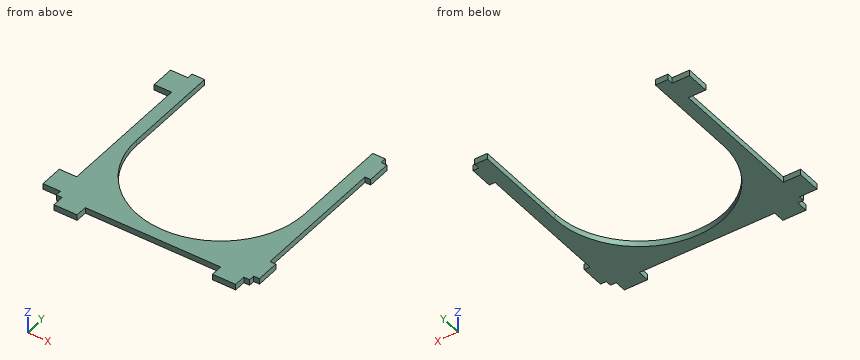
```python
from build123d import *

# Parameters (mm, degrees)
CROQUIS1_W              = 100
CROQUIS1_H              = 100
CROQUIS1_R              = 43.5
SALIENTE_EXTRUIR1_DEPTH = 3
CROQUIS2_W              = 12
CROQUIS2_H              = 6
CROQUIS2_W_2            = 9
CROQUIS2_H_2            = 12
CROQUIS2_W_3            = 3
SALIENTE_EXTRUIR2_DEPTH = 3
CROQUIS3_W              = 87
CROQUIS3_H              = 50
CORTAR_EXTRUIR1_DEPTH   = 10


with BuildPart() as part:
    # Croquis1 → Saliente-Extruir1 (new body)
    with BuildSketch(Plane.XY):
        Rectangle(CROQUIS1_W, CROQUIS1_H)
        Circle(CROQUIS1_R, mode=Mode.SUBTRACT)
    extrude(amount=SALIENTE_EXTRUIR1_DEPTH)

    # Croquis2 → Saliente-Extruir2 (add)
    with BuildSketch(Plane.XY.offset(3)):
        with Locations((-41, -53)):
            Rectangle(CROQUIS2_W, CROQUIS2_H)
        with Locations((41, -53)):
            Rectangle(CROQUIS2_W, CROQUIS2_H)
        with Locations((-54.5, -41)):
            Rectangle(CROQUIS2_W_2, CROQUIS2_H_2)
        with Locations((51.5, -41)):
            Rectangle(CROQUIS2_W_3, CROQUIS2_H_2)
        with Locations((51.5, 41)):
            Rectangle(CROQUIS2_W_3, CROQUIS2_H_2)
        with Locations((-54.5, 41)):
            Rectangle(CROQUIS2_W_2, CROQUIS2_H_2)
    extrude(amount=-SALIENTE_EXTRUIR2_DEPTH)

    # Croquis3 → Cortar-Extruir1 (cut)
    with BuildSketch(Plane.XY.offset(3)):
        with Locations((0, 25)):
            Rectangle(CROQUIS3_W, CROQUIS3_H)
    extrude(amount=-CORTAR_EXTRUIR1_DEPTH, mode=Mode.SUBTRACT)


solid = part.part
```
Geometry: final body of the model. Coordinates: model frame, mm. Round coordinates to 2 decimals unless told otherwise and drop trailing zeros. Order: outer loops, then holes, each group sorted by start corner. A loop starts at its lowest first (then second) coordinate and runs counter-clockwise, first axis right, second up. Notation, with made-up numbers: (-17.5, -19) - (34.5, -19) arc R12 ccw to (34.5, -6) - close; hole circle Ø6 at (37, -19.75). An arc over 180 degrees is marked (long way). Write item = value, one per line. Start each with the question number.
Q1. Cut plane C-C on x = 0. Return the cut outline in (y, z), and give its area (3 significant figures).
Q2. Cut plane A-A on y = 10. Return the cut outline in (x, z).
Q3. Ray query, line 1 (X direction, y = 15, z = 1.4); line 2 (Y direction, x = -54, z = 0.3); line 3 (Y direction, x = -1.5, z = 0.4). Return the intervals inside material, ascending. Write a range as from..to.
Q4. Cut plane D-D on x = 26. Return the cut outline in (y, z), and give its area (3 significant figures).
Q5. Pin query (flat end, axial travel): pin 1 (0.9 mm diameter, centred on x = -53, z = 1.5, fed in from +Y); pin 2 (2 mm diameter, centred on x = -46, y = 32, fed in from -Z); pin 3 (1.5 mm diameter, centred on x = 51.5, z = 1.5, fed in from -Y); pin 4 (1.5 mm diameter, centred on y = -48, z = 1.5, fed in from +X). Return the tip coordinate at first contact, or that it passes through.
Outcome:
q1.outline = (-50, 0) - (-43.5, 0) - (-43.5, 3) - (-50, 3) - close
q1.area = 19.5 mm^2
q2.outline = (-50, 0) - (-43.5, 0) - (-43.5, 3) - (-50, 3) - close; (43.5, 0) - (50, 0) - (50, 3) - (43.5, 3) - close
q3.line_1 = -50..-43.5, 43.5..50
q3.line_2 = -47..-35, 35..47
q3.line_3 = -50..-43.47
q4.outline = (-50, 0) - (-34.87, 0) - (-34.87, 3) - (-50, 3) - close
q4.area = 45.4 mm^2
q5.pin_1 = 47
q5.pin_2 = 0
q5.pin_3 = -47
q5.pin_4 = 50
